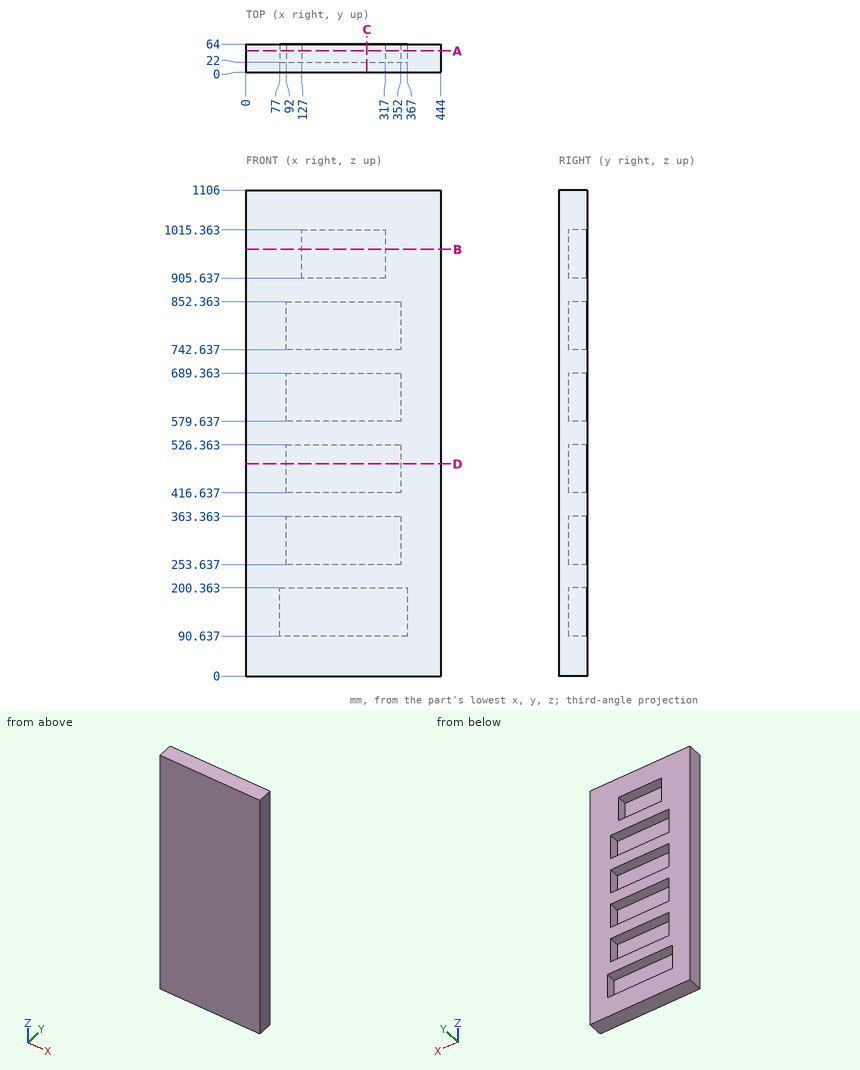
Source: three-view drawing plus pictorial views. Frame: mm from the lowest corner of the part. Coordinates: 2 decimals unless noted, no trailing zeros. Write each loop counter-clockwise with the first axis right and the second up, starting at its lowest first coordinate (ties: lowest second). Pieces come first, ordered by that corner, then holes. Notation, with made-up numbers: (70, 66) - (116, 66) arc R9 cw to (116, 82) - close; hole circle Ø3 at (56.25, 72.5). An arc over 180 degrees is marked (long way). Return JSON: item names as keys, results as strings.
Item 1: Section query B-B (z = 971). Output: boundary loops of the cut face in (x, y).
Completed:
{"outline": "(0, 0) - (444, 0) - (444, 64) - (317, 64) - (317, 22) - (127, 22) - (127, 64) - (0, 64) - close"}
Item 2: Section query C-C (x = 275.5). Output: boundary loops of the cut face in (y, z).
Completed:
{"outline": "(0, 0) - (64, 0) - (64, 90.64) - (22, 90.64) - (22, 200.36) - (64, 200.36) - (64, 253.64) - (22, 253.64) - (22, 363.36) - (64, 363.36) - (64, 416.64) - (22, 416.64) - (22, 526.36) - (64, 526.36) - (64, 579.64) - (22, 579.64) - (22, 689.36) - (64, 689.36) - (64, 742.64) - (22, 742.64) - (22, 852.36) - (64, 852.36) - (64, 905.64) - (22, 905.64) - (22, 1015.36) - (64, 1015.36) - (64, 1106) - (0, 1106) - close"}
Item 3: Pin query (flat end, axial travel): pin 1 Ø6 at (x, z) = (330.5, 307) entering from +Y. Return the tip coordinate at first contact, or that it passes through.
Completed:
{"pin 1": "stops at y = 22"}
Item 4: Section query D-D (z = 483). Output: boundary loops of the cut face in (x, y), and give its area (3 significant figures).
Completed:
{"outline": "(0, 0) - (444, 0) - (444, 64) - (352, 64) - (352, 22) - (92, 22) - (92, 64) - (0, 64) - close", "area": "17,500 mm2"}
Item 5: Line query: L1, parallel to Z at x = 340, y = 32.5; L2, parallel to X at y = 35.5, z = 812; L3, parallel to Z at x = 357, y = 34. Output: solid intervals per line, ascending.
Completed:
{"L1": "z = 0 to 90.64, 200.36 to 253.64, 363.36 to 416.64, 526.36 to 579.64, 689.36 to 742.64, 852.36 to 1106", "L2": "x = 0 to 92, 352 to 444", "L3": "z = 0 to 90.64, 200.36 to 1106"}
Item 6: Section query A-A (y = 48.5). Output: boundary loops of the cut face in (x, z).
Completed:
{"outline": "(0, 0) - (444, 0) - (444, 1106) - (0, 1106) - close; hole (77, 90.64) - (367, 90.64) - (367, 200.36) - (77, 200.36) - close; hole (92, 253.64) - (352, 253.64) - (352, 363.36) - (92, 363.36) - close; hole (92, 416.64) - (352, 416.64) - (352, 526.36) - (92, 526.36) - close; hole (92, 579.64) - (352, 579.64) - (352, 689.36) - (92, 689.36) - close; hole (92, 742.64) - (352, 742.64) - (352, 852.36) - (92, 852.36) - close; hole (127, 905.64) - (317, 905.64) - (317, 1015.36) - (127, 1015.36) - close"}
